Here's how the part is built. I have some questions about the finished solid (model axes, mm). A direction names the side the tool comes from. Round coordinates to 2 decimals unless told otherwise and drop trailing zeros. Write each loop counter-clockwise with the first axis right and the second up, starting at its lowest first coordinate (ties: lowest second). Pieces come first, ordered by that corner, then holes. Notation, with made-up numbers: (-17.75, 53) - (40.25, 53) arc R30 ccw to (40.25, 87) - close; hole circle Ø10 at (48.25, 70). An arc over 180 degrees is marked (long way). Write item = value, one per line. Start each with the question number.
Item 1: Thinking about a two-plate mould opening in Z: for faces 3 (the face through (110.961, 2.415, -92.695)), 4 (the face through (-1.6, 2.35, 152.39)), 5 (the face through (1.6, 2.35, -152.39)), which applies, pulls with the +Z half, pulls with the -Z half, needs draft (parallel to the pull), parting line crosses it, or undercut?
Item 2: For P1, Ø2.5, axis at x = 15, z = 15, coming from the -Y side; P2, Ø2, axis at y = 1, z = 17, coming from the +X side; P3, Ø1.5, axis at x = 22, y = 3.5, coming from the +Z side, each with a flat end and sliding along its axis, tell me the tip position at first contact or that it passes through.
Item 3: If we section it at A-A (y = 3.35): Give the number of separate pieces and of enclosed holes in the cut face, and give its area (3 significant figures).
Item 4: Which directions (+Z, -Z, +X, -X, +Y, -Y) give clear straight access to the entire face, cutting with the end or side of a thin tool? Please do faces 1 (the face through (-152.39, 2.35, -1.6)), 2 (the face through (-30.442, 2.415, -29.203)).
Item 5: If I drill on line 1 along Z through (x, y) = (85, 0.2); line 2 along X through (y, z) = (0.9, 63); line 3 along X through (y, z) = (3.9, 73), over which ranges is the centre line in solid material (lowest first)? Write a range as [from, to].
Item 6: If we section it at B-B (x = -56): Please give me the cut outline in (y, z).
Item 7: If we section it at C-C (z = -56): Please give me the cut outline in (x, y), and give its area (3 significant figures).
```python
from build123d import *

# Parameters (mm, degrees)
SKETCH1_R                = 152.4
BOSS_EXTRUDE1_DEPTH      = 4.7625
F_8_CLEARANCE_HOLE1_D    = 4.4958
CIRPATTERN1_COUNT        = 12
M2_5_CLEARANCE_HOLE1_D   = 2.9
CUT_EXTRUDE1_DEPTH       = 216.578759172
FILLET1_R                = 3
FILLET2_R                = 2
FILLET3_R                = 8
CIRPATTERN2_COUNT        = 4
FILLET1_OF_CIRPATTERN2_R = 3
FILLET2_OF_CIRPATTERN2_R = 2
FILLET3_OF_CIRPATTERN2_R = 8
M5_CLEARANCE_HOLE1_D     = 5.5
M5_CLEARANCE_HOLE2_D     = 5.5
CIRPATTERN3_COUNT        = 12
CUT_EXTRUDE3_REACH       = 217.579
SKETCH15_R               = 9.525
CUT_EXTRUDE4_REACH       = 217.579


with BuildPart() as part:
    # Sketch1 → Boss-Extrude1 (new body)
    with BuildSketch(Plane(origin=(0, 0, 0), x_dir=(1, 0, 0), z_dir=(0, 1, 0))):
        with Locations(Location((0, 0, 0), (0, 0, 90))):
            Circle(SKETCH1_R)
    extrude(amount=BOSS_EXTRUDE1_DEPTH)

    # #8 Clearance Hole1 (through all)
    with Locations(Plane(origin=(0, 4.7625, 0), x_dir=(1, 0, 0), z_dir=(0, 1, 0))):
        with Locations((0, -142.875)):
            f_8_clearance_hole1 = Hole(F_8_CLEARANCE_HOLE1_D / 2)

    # CirPattern1: #8 Clearance Hole1 ×12 about axis
    cirpattern1_axis = Axis((0, 0, 0), (0, 1, 0))
    for i in range(1, CIRPATTERN1_COUNT):
        add(f_8_clearance_hole1.rotate(cirpattern1_axis, i * 360 / CIRPATTERN1_COUNT), mode=Mode.SUBTRACT)

    # M2.5 Clearance Hole1 (through all)
    with Locations(Plane(origin=(0, 4.7625, 0), x_dir=(1, 0, 0), z_dir=(0, 1, 0))):
        with Locations((-15, -15), (-15, 15), (15, 15), (15, -15)):
            Hole(M2_5_CLEARANCE_HOLE1_D / 2)

    # Sketch8 → Cut-Extrude1 (cut, through all)
    with BuildSketch(Plane(origin=(0, 4.7625, 0), x_dir=(1, 0, 0), z_dir=(0, 1, 0))):
        Polygon((105.641753109, -109.884393796), (95.464119439, -99.706760126), (86.978838065, -108.192041501), (82.736197378, -103.949400814), (95.464119439, -91.221478752), (109.884393796, -105.641753109), align=None)
        with BuildLine():
            Line((86.271731284, -113.141788969), (94.757012658, -104.656507595))
            ThreePointArc((94.757012658, -104.656507595), (96.878333002, -104.656507595), (96.878333002, -106.777827938))
            Line((96.878333002, -106.777827938), (88.393051627, -115.263109313))
            ThreePointArc((88.393051627, -115.263109313), (86.271731284, -115.263109313), (86.271731284, -113.141788969))
        make_face()
        with BuildLine():
            Line((77.78644991, -104.656507595), (86.271731284, -96.17122622))
            ThreePointArc((86.271731284, -96.17122622), (86.271731284, -94.049905877), (84.15041094, -94.049905877))
            Line((84.15041094, -94.049905877), (75.665129566, -102.535187251))
            ThreePointArc((75.665129566, -102.535187251), (75.665129566, -104.656507595), (77.78644991, -104.656507595))
        make_face()
    cut_extrude1 = extrude(amount=-CUT_EXTRUDE1_DEPTH, mode=Mode.SUBTRACT)

    # Fillet1
    fillet1_edges = [part.edges().sort_by_distance(p)[0] for p in [
        (86.978838065, 2.38125, 108.192041501),
        (82.736197378, 2.38125, 103.949400814),
    ]]
    fillet(fillet1_edges, radius=FILLET1_R - 0.0001)  # a hair under: the kernel refuses the full size

    # Fillet2
    fillet2_edges = [part.edges().sort_by_distance(p)[0] for p in [
        (105.620871949, 2.38125, 109.863512636),
        (109.863512636, 2.38125, 105.620871949),
        (95.464119439, 2.38125, 99.706760126),
    ]]
    fillet(fillet2_edges, radius=FILLET2_R)

    # Fillet3
    fillet3_edges = [part.edges().sort_by_distance(p)[0] for p in [
        (95.464119439, 2.38125, 91.221478752),
    ]]
    fillet(fillet3_edges, radius=FILLET3_R)

    # CirPattern2: Cut-Extrude1 ×4 about axis
    cirpattern2_axis = Axis((0, 0, 0), (0, 1, 0))
    for i in range(1, CIRPATTERN2_COUNT):
        add(cut_extrude1.rotate(cirpattern2_axis, i * 360 / CIRPATTERN2_COUNT), mode=Mode.SUBTRACT)

    # Fillet1 of CirPattern2
    fillet1_of_cirpattern2_edges = [part.edges().sort_by_distance(p)[0] for p in [
        (108.192041501, 2.38125, -86.978838065),
        (103.949400814, 2.38125, -82.736197378),
        (-86.978838065, 2.38125, -108.192041501),
        (-82.736197378, 2.38125, -103.949400814),
        (-108.192041501, 2.38125, 86.978838065),
        (-103.949400814, 2.38125, 82.736197378),
    ]]
    fillet(fillet1_of_cirpattern2_edges, radius=FILLET1_OF_CIRPATTERN2_R - 0.0001)  # a hair under: the kernel refuses the full size

    # Fillet2 of CirPattern2
    fillet2_of_cirpattern2_edges = [part.edges().sort_by_distance(p)[0] for p in [
        (109.863512636, 2.38125, -105.620871949),
        (105.620871949, 2.38125, -109.863512636),
        (99.706760126, 2.38125, -95.464119439),
        (-105.620871949, 2.38125, -109.863512636),
        (-109.863512636, 2.38125, -105.620871949),
        (-95.464119439, 2.38125, -99.706760126),
        (-109.863512636, 2.38125, 105.620871949),
        (-105.620871949, 2.38125, 109.863512636),
        (-99.706760126, 2.38125, 95.464119439),
    ]]
    fillet(fillet2_of_cirpattern2_edges, radius=FILLET2_OF_CIRPATTERN2_R)

    # Fillet3 of CirPattern2
    fillet3_of_cirpattern2_edges = [part.edges().sort_by_distance(p)[0] for p in [
        (91.221478752, 2.38125, -95.464119439),
        (-95.464119439, 2.38125, -91.221478752),
        (-91.221478752, 2.38125, 95.464119439),
    ]]
    fillet(fillet3_of_cirpattern2_edges, radius=FILLET3_OF_CIRPATTERN2_R)

    # M5 Clearance Hole1 (through all)
    with Locations(Plane(origin=(0, 4.7625, 0), x_dir=(1, 0, 0), z_dir=(0, 1, 0))):
        with Locations((-13.2, -35.21), (13.2, -35.21), (27.62, -64.79), (13.2, -94.36), (-13.2, -94.36), (-27.62, -64.79)):
            Hole(M5_CLEARANCE_HOLE1_D / 2)

    # M5 Clearance Hole2 (through all)
    with Locations(Plane(origin=(0, 4.7625, 0), x_dir=(1, 0, 0), z_dir=(0, 1, 0))):
        with Locations((32.354102414, -120.747154041), (37.685774743, -140.645226063)):
            m5_clearance_hole2 = Hole(M5_CLEARANCE_HOLE2_D / 2)

    # CirPattern3: M5 Clearance Hole2 ×12 about axis, 4 skipped
    cirpattern3_axis = Axis((0, 0, 0), (0, -1, 0))
    add([m5_clearance_hole2.rotate(cirpattern3_axis, i * 360 / CIRPATTERN3_COUNT) for i in range(1, CIRPATTERN3_COUNT) if i not in (2, 5, 8, 11)], mode=Mode.SUBTRACT)

    # Sketch15 → Cut-Extrude3 (cut, up to next)
    with BuildSketch(Plane(origin=(0, 4.7625, 0), x_dir=(1, 0, 0), z_dir=(0, 1, 0)), mode=Mode.PRIVATE) as cut_extrude3_sk1:
        with Locations(Location((-1.242160376, 87.572306541, 0), (0, 0, 270))):
            Circle(SKETCH15_R)
    cut_extrude3_tool1 = extrude(cut_extrude3_sk1.sketch, amount=-CUT_EXTRUDE3_REACH, mode=Mode.PRIVATE) & part.part
    add(cut_extrude3_tool1.solids().sort_by_distance((-1.24216, 4.7625, -87.572307))[0], mode=Mode.SUBTRACT)

    # Sketch16 → Cut-Extrude4 (cut, up to next)
    with BuildSketch(Plane(origin=(0, 4.7625, 0), x_dir=(1, 0, 0), z_dir=(0, 1, 0)), mode=Mode.PRIVATE) as cut_extrude4_sk1:
        Polygon((40.769638118, 23.532806086), (34.565538825, 12.232482372), (13.617375959, 23.733434534), (19.821475253, 35.033758247), align=None)
    cut_extrude4_tool1 = extrude(cut_extrude4_sk1.sketch, amount=-CUT_EXTRUDE4_REACH, mode=Mode.PRIVATE) & part.part
    # Sketch16 → Cut-Extrude4 (cut, up to next)
    with BuildSketch(Plane(origin=(0, 4.7625, 0), x_dir=(1, 0, 0), z_dir=(0, 1, 0)), mode=Mode.PRIVATE) as cut_extrude4_sk2:
        Polygon((-19.821475253, 35.033758247), (-13.617375959, 23.733434534), (-34.565538825, 12.232482372), (-40.769638118, 23.532806086), align=None)
    cut_extrude4_tool2 = extrude(cut_extrude4_sk2.sketch, amount=-CUT_EXTRUDE4_REACH, mode=Mode.PRIVATE) & part.part
    add(cut_extrude4_tool1.solids().sort_by_distance((27.193507, 4.7625, -23.63312))[0], mode=Mode.SUBTRACT)
    add(cut_extrude4_tool2.solids().sort_by_distance((-27.193507, 4.7625, -23.63312))[0], mode=Mode.SUBTRACT)


solid = part.part
```
Reply:
q1.face_3 = undercut
q1.face_4 = pulls with the +Z half
q1.face_5 = pulls with the -Z half
q2.P1 = through
q2.P2 = 151.56
q2.P3 = 150.91
q3.separate_pieces = 1
q3.enclosed_holes = 49
q3.area = 70,300 mm2
q4.face_1 = -X, +Y, -Y
q4.face_2 = +Y, -Y
q5.line_1 = [-126.49, 93.63], [97.44, 101.69], [106.2, 126.49]
q5.line_2 = [-138.77, -29.71], [-25.53, 25.53], [29.71, 138.77]
q5.line_3 = [-133.78, -125.35], [-122.12, 122.12], [125.35, 133.78]
q6.outline = (0, -141.74) - (4.76, -141.74) - (4.76, 141.74) - (0, 141.74) - close
q7.outline = (-141.74, 0) - (141.74, 0) - (141.74, 4.76) - (-141.74, 4.76) - close
q7.area = 1,350 mm2
